```python
from build123d import *

# Parameters (mm, degrees)
SKETCH_1_W      = 110
SKETCH_1_H      = 80
EXTRUDE_1_DEPTH = 6
EXTRUDE_2_DEPTH = 6


with BuildPart() as part:
    # Эскиз1 → Бобышка-Вытянуть1 (new body)
    with BuildSketch(Plane.XY):
        Rectangle(SKETCH_1_W, SKETCH_1_H)
    extrude(amount=EXTRUDE_1_DEPTH)

    # Эскиз2 → Бобышка-Вытянуть2 (add)
    with BuildSketch(Plane.XY.offset(6)):
        with BuildLine():
            Line((124.05, 82.05), (42, 82.05))
            Line((42, 82.05), (42, -82.05))
            Line((42, -82.05), (124.05, -82.05))
            Line((124.05, -82.05), (124.05, -69.05))
            ThreePointArc((124.05, -69.05), (55, 0), (124.05, 69.05))
            Line((124.05, 69.05), (124.05, 82.05))
        make_face()
    extrude(amount=-EXTRUDE_2_DEPTH)


solid = part.part
```
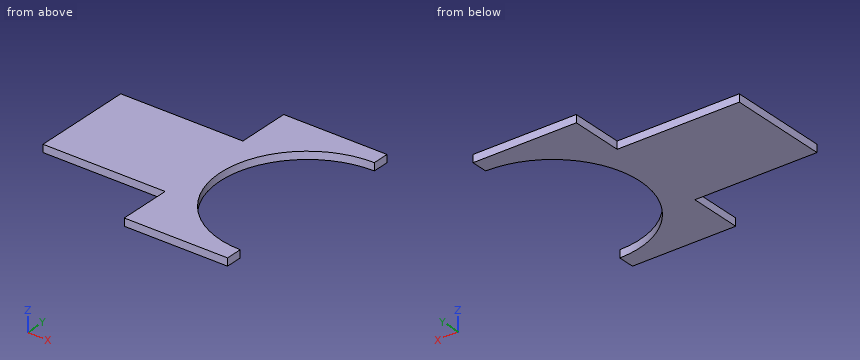
Work out the finished part from the listing and answer in its coordinate system (mm). Give positions to 0.01 mm unless a question says otherwise; leave off trailing zeros. Write each loop counter-clockwise with the first axis right and the second up, starting at its lowest first coordinate (ties: lowest second). Pieces come first, ordered by that corner, then holes. Notation, with made-up numbers: (48, 66) -> (87, 66) arc R23 ccw to (87, 103) -> close; hole circle Ø1 at (79.5, 3). An arc over 180 degrees is marked (long way). Write item = value, one per line.
Q1. Section C-C on y = 0 is taken. Determine the outline of the cut face in (x, z).
Computed values:
outline = (-55, 0) -> (55, 0) -> (55, 6) -> (-55, 6) -> close
Q2. Section A-A on z = 2.2 is taken. Determine the outline of the cut face in (x, y), and give its area (3 significant figures).
Computed values:
outline = (-55, -40) -> (42, -40) -> (42, -82.05) -> (124.05, -82.05) -> (124.05, -69.05) arc R69.05 cw to (124.05, 69.05) -> (124.05, 82.05) -> (42, 82.05) -> (42, 40) -> (-55, 40) -> close
area = 13,700 mm^2
Q3. Section B-B on x = 57 is taken. Determine the outline of the cut face in (y, z).
Computed values:
outline = (-82.05, 0) -> (-16.5, 0) -> (-16.5, 6) -> (-82.05, 6) -> close; (16.5, 0) -> (82.05, 0) -> (82.05, 6) -> (16.5, 6) -> close
Q4. Section D-D on x = 109 is taken. Determine the outline of the cut face in (y, z), and give its area (3 significant figures).
Computed values:
outline = (-82.05, 0) -> (-67.39, 0) -> (-67.39, 6) -> (-82.05, 6) -> close; (67.39, 0) -> (82.05, 0) -> (82.05, 6) -> (67.39, 6) -> close
area = 176 mm^2
Q5. Consider line 1 along Y through (x, z) = (-33.5, 3.55); line 2 along X through (y, z) = (-72, 4.85); line 3 along Y through (x, z) = (64, 5.75). Determine where each line is inside the solid, lowest interval first.
Computed values:
line_1 = -40 to 40
line_2 = 42 to 124.05
line_3 = -82.05 to -34.09, 34.09 to 82.05
Q6. Flat-ended cylindrical pins translate along their axes: pin 1 Ø3 at (y, z) = (-44.5, 5) entering from -X; pin 2 Ø3 at (x, z) = (-26.5, 2) entering from -Y; pin 3 Ø3 at (x, z) = (27, 1) entering from +Y. Find the tip coordinate at first contact, or state that the pin passes through.
Computed values:
pin_1 = 42
pin_2 = -40
pin_3 = 40
